Check sheet for the modelled part. Datum: model origin and axes. Units: mm. A direction names the side the tool comes from. Give positions to 0.01 mm unless a question says otherwise; leave off trailing zeros. Order: outer loops, then holes, each group sorted by start corner. A loop starts at its lowest first (then second) coordinate and runs counter-clockwise, first axis right, second up. Notation, with made-up numbers: M 4,33 L 27,33 A16 cw 27,56 Z; hole C -24.75,34.5 d11. An arc over 180 degrees is marked long. Return JSON: item names as keys, results as strings. Group by question number.
Autodesk Inventor part; units mm, degrees
ref_plane "YZ Plane" through (0, 0, 0) normal (1, 0, 0) x (0, 1, 0)
ref_plane "XZ Plane" through (0, 0, 0) normal (0, 1, 0) x (-1, 0, 0)
ref_plane "XY Plane" through (0, 0, 0) normal (0, 0, 1) x (1, 0, 0)
sketch "Sketch51" plane through (0, 0, 0) normal (0, 1, 0) x (-1, 0, 0)
  line L0 (1.3484, 37.0338) -> (-3.7316, 37.0338)
  line L1 (-3.7316, 37.0338) -> (-3.7316, -191.5662)
  line L2 (-3.7316, -191.5662) -> (1.3484, -191.5662)
  line L3 (1.3484, -191.5662) -> (1.3484, 37.0338)
  point P0 (0, 0)
  dimension "d172" = 5.08
  dimension "d173" = 228.6
extrude "Extrusion37" add sketch "Sketch51" along normal blind 71.12
sketch "Sketch52" plane through (-1.3484, 0, 37.0338) normal (0, 0, 1) x (1, 0, 0)
  line L0 (5.08, 0) -> (5.08, 71.12)
  line L1 (5.08, 71.12) -> (-24.13, 71.12)
  line L2 (-24.13, 71.12) -> (-24.13, 66.04)
  line L3 (-24.13, 66.04) -> (5.08, 66.04)
  line L4 (5.08, 66.04) -> (5.08, 71.12)
  point P0 (1.3484, 0)
  dimension "d176" = 5.08
  dimension "d177" = 29.21
extrude "Extrusion38" add sketch "Sketch52" against normal blind 228.6
sketch "Sketch54" plane through (0, 0, 0) normal (0, -1, 0) x (1, 0, 0)
  line L0 (-20.3984, 37.0338) -> (-141.0484, 37.0338)
  line L1 (-141.0484, 37.0338) -> (-141.0484, -191.5662)
  line L2 (-141.0484, -191.5662) -> (-20.3984, -191.5662)
  line L3 (-20.3984, -191.5662) -> (-20.3984, 37.0338)
  line L4 (-25.4784, 37.0338) -> (-1.3484, 37.0338)
  line L5 (-1.3484, -191.5662) -> (-25.4784, -191.5662)
  line L6 (-1.3484, -191.5662) -> (-1.3484, 37.0338)
  point P0 (0, 0)
  dimension "d180" = 0
  dimension "d181" = 0
  dimension "d182" = 19.05
  dimension "d183" = 120.65
extrude "Extrusion39" add sketch "Sketch54" against normal blind 5.08 contours L3 L2 L1 L0
sketch "Sketch55" plane through (-1.3484, 0, 37.0338) normal (0, 0, 1) x (1, 0, 0)
  line L0 (-139.7, 5.08) -> (-19.05, 5.08)
  line L1 (-24.13, 66.04) -> (-24.13, 71.12)
  line L2 (-19.05, 5.08) -> (-24.13, 5.08)
  line L3 (-24.13, 5.08) -> (-24.13, 71.12)
  line L4 (-24.13, 71.12) -> (-19.05, 71.12)
  line L5 (-19.05, 71.12) -> (-19.05, 5.08)
  point P0 (1.3484, 0)
extrude "Extrusion40" add sketch "Sketch55" against normal blind 228.6
sketch "Sketch56" plane through (3.7316, 0, 37.0338) normal (0, 0, 1) x (1, 0, 0)
  line L0 (-29.4089, 71.1531) -> (0, 71.1531)
  line L1 (0, 71.1531) -> (0, 0)
  line L2 (0, 0) -> (-29.4089, 0)
  line L3 (-29.4089, 0) -> (-29.4089, 71.1531)
  point P0 (-3.7316, 0)
extrude "Extrusion41" add sketch "Sketch56" against normal blind 5.08
sketch "Sketch57" plane through (3.7316, 0, -191.5662) normal (0, 0, -1) x (-1, 0, 0)
  line L0 (29.4089, 5.08) -> (29.4089, 71.1531)
  line L1 (29.4089, 71.1531) -> (0, 71.1531)
  line L2 (0, 71.1531) -> (0, 0)
  line L3 (0, 0) -> (29.4089, 0)
  line L4 (29.4089, 0) -> (29.4089, 71.1531)
  point P0 (3.7316, 0)
extrude "Extrusion42" add sketch "Sketch57" against normal blind 5.08
sketch "Sketch58" plane through (0, 71.12, 0) normal (0, 1, 0) x (1, 0, 0)
  line L0 (-25.4784, -31.9538) -> (-25.4784, 186.4862)
  line L1 (-141.0484, 191.5662) -> (-141.0484, -37.0338)
  line L2 (-25.4784, 109.0162) -> (-141.0484, 109.0162)
  line L3 (-141.0484, 109.0162) -> (-141.0484, 147.1162)
  line L4 (-141.0484, 147.1162) -> (-25.4784, 147.1162)
  line L5 (-25.4784, 147.1162) -> (-25.4784, 109.0162)
  line L6 (-25.6773, 191.5662) -> (-141.0484, 191.5662)
  point P0 (0, 0)
  dimension "d192" = 38.1
  dimension "d193" = 44.45
extrude "Extrusion43" add sketch "Sketch58" against normal blind 5.08
sketch "Sketch59" plane through (-141.0484, 71.12, -147.1162) normal (-1, 0, 0) x (0, 0, 1)
  line L0 (0, 0) -> (0, -5.08)
  line L1 (184.15, -71.12) -> (-44.45, -71.12)
  line L2 (0, 0) -> (5.08, 0)
  line L3 (5.08, 0) -> (5.08, -71.12)
  line L4 (5.08, -71.12) -> (0, -71.12)
  line L5 (0, -71.12) -> (0, 0)
  line L6 (38.1, 0) -> (38.1, -5.08)
  line L7 (38.1, 0) -> (33.02, 0)
  line L8 (33.02, 0) -> (33.02, -71.12)
  line L9 (33.02, -71.12) -> (38.1, -71.12)
  line L10 (38.1, -71.12) -> (38.1, 0)
  point P0 (147.1162, -71.12)
  dimension "d196" = 5.08
  dimension "d197" = 5.08
extrude "Extrusion44" add sketch "Sketch59" against normal blind 120.65
sketch "Sketch60" plane through (-141.0484, 0, -191.5662) normal (-1, 0, 0) x (0, 0, 1)
  line L0 (49.53, 5.08) -> (77.47, 5.08)
  line L1 (5.08, 0) -> (223.52, 0)
  line L2 (49.53, 5.08) -> (77.4104, 5.08)
  line L3 (77.4104, 5.08) -> (77.4104, 0)
  line L4 (77.4104, 0) -> (49.53, 0)
  line L5 (49.53, 0) -> (49.53, 5.08)
  point P0 (191.5662, 0)
extrude "Extrusion45" cut sketch "Sketch60" against normal blind 120.65
sketch "Sketch61" plane through (-25.4784, 66.04, -142.0362) normal (-1, 0, 0) x (0, 0, 1)
  line L0 (0, -66.04) -> (0, 0)
  line L1 (27.94, 0) -> (27.94, -60.96)
  line L2 (27.94, 0) -> (0, 0)
  line L3 (-44.45, -66.04) -> (173.99, -66.04)
  line L4 (0, 0) -> (27.6512, 0)
  line L5 (27.6512, 0) -> (27.6512, -66.04)
  line L6 (27.6512, -66.04) -> (0, -66.04)
  line L7 (0, -66.04) -> (0, 0)
  point P0 (142.0362, -66.04)
extrude "Extrusion46" cut sketch "Sketch61" against normal blind 5.08
sketch "Sketch62" plane through (-141.0484, 5.08, -109.0162) normal (-1, 0, 0) x (0, 0, 1)
  line L0 (-33.02, -5.08) -> (-82.55, -5.08)
  line L1 (-38.1, 66.04) -> (-38.1, 0)
  line L2 (0, 66.04) -> (0, 0)
  line L3 (-5.1396, 0) -> (-5.1396, -5.08)
  line L4 (146.05, -5.08) -> (-5.1396, -5.08)
  line L5 (146.05, -5.08) -> (146.05, 0)
  line L6 (0, 0) -> (146.05, 0)
  line L7 (0, 66.04) -> (0, 0)
  line L8 (0, 66.04) -> (-38.1, 66.04)
  line L9 (-38.1, 66.04) -> (-38.1, 0)
  line L10 (-82.55, 0) -> (-38.1, 0)
  line L11 (-82.55, -5.08) -> (-82.55, 0)
  line L12 (-33.02, -5.08) -> (-82.55, -5.08)
  line L13 (-33.02, -5.08) -> (-33.02, 60.96)
  line L14 (-5.08, 60.96) -> (-33.02, 60.96)
  line L15 (-5.08, 60.96) -> (-5.08, 0)
  line L16 (0, 66.04) -> (-34.1859, 66.04)
  line L17 (-34.1859, 66.04) -> (-34.1859, -5.08)
  line L18 (-34.1859, -5.08) -> (0, -5.08)
  line L19 (0, -5.08) -> (0, 66.04)
  line L20 (-5.1396, 0) -> (-5.08, 0)
  point P0 (109.0162, -5.08)
extrude "Extrusion47" add sketch "Sketch62" against normal blind 5.08 contours L0 L17 L8 L2 L19 L4 L3 L20 L15 L14 L13 | L13 L14 L15 L20 L3 L18
sketch "Sketch63" plane through (3.7316, 0, -191.5662) normal (0, 0, -1) x (-1, 0, 0)
  line L0 (0, 0) -> (144.78, 0)
  line L1 (29.4089, 5.08) -> (29.4089, 71.1531)
  point P0 (3.7316, 0)
  point P1 (14.1689, 25.4)
  dimension "d206" = 25.4
  dimension "d207" = 15.24
hole "Hole8" at (-10.4373, 25.4, -191.5662) direction (0, 0, 1) diameter 3.302 end through all
sketch "Sketch64" plane through (-141.0484, 0, -191.5662) normal (-1, 0, 0) x (0, 0, 1)
  line L0 (228.6, 0) -> (0, 0)
  line L1 (44.45, 71.12) -> (44.45, 5.08)
  point P0 (191.5662, 0)
  point P1 (63.5, 25.4)
  dimension "d215" = 25.4
  dimension "d216" = 19.05
hole "Hole9" at (-141.0484, 25.4, -128.0662) direction (1, 0, 0) diameter 3.302 depth 25.4 tip angle 118.188
sketch "Sketch66" plane through (0, 71.12, 0) normal (0, 1, 0) x (1, 0, 0)
  line L0 (-141.0484, 109.0162) -> (-141.0484, 147.1162)
  line L1 (-25.4784, 109.0162) -> (-141.0484, 109.0162)
  line L2 (-141.0484, 147.1162) -> (-25.4784, 147.1162)
  point P0 (0, 0)
  point P1 (-77.5484, 137.5912)
  point P2 (-77.5484, 118.5412)
  dimension "d224" = 0
  dimension "d225" = 63.5
  dimension "d226" = 9.525
  dimension "d227" = 9.525
hole "Hole10" at (-77.5484, 71.12, -137.5912) at (-77.5484, 71.12, -118.5412) direction (0, -1, 0) diameter 3.81 depth 25.4 tip angle 118.188
sketch "Sketch67" plane through (0, 71.12, 0) normal (0, 1, 0) x (1, 0, 0)
  line L0 (-25.4784, -31.9538) -> (-25.4784, 109.0162)
  line L1 (-25.6773, -37.0338) -> (3.7316, -37.0338)
  point P0 (0, 0)
  point P1 (-10.8734, -24.3338)
  point P2 (-10.8734, 51.8662)
  dimension "d235" = 0
  dimension "d236" = 76.2
  dimension "d237" = 14.605
  dimension "d238" = 12.7
hole "Hole11" at (-10.8734, 71.12, 24.3338) at (-10.8734, 71.12, -51.8662) direction (0, -1, 0) diameter 3.81 depth 25.4 tip angle 118.188
sketch "Sketch68" plane through (-141.0484, 71.12, -109.0162) normal (0, 0, 1) x (1, 0, 0)
  line L0 (50.8, -38.1) -> (76.2, -38.1) construction
  line L1 (50.8, -63.5) -> (76.2, -63.5)
  line L2 (76.2, -12.7) -> (50.8, -12.7)
  arc A0 (50.8, -12.7) -> (50.8, -63.5) centre (50.8, -38.1) ccw
  arc A1 (76.2, -63.5) -> (76.2, -12.7) centre (76.2, -38.1) ccw
  line L3 (115.57, 0) -> (0, 0)
  line L4 (0, 0) -> (0, -66.04)
  point P0 (141.0484, -71.12)
  point P1 (63.5, -38.1)
  dimension "d246" = 38.1
  dimension "d247" = 25.4
  dimension "d248" = 50.8
  dimension "d249" = 25.4
extrude "Extrusion48" cut sketch "Sketch68" against normal blind 77.7875
equation "\"d172\" = WallWidth"
equation "\"d173\" = PartLength"
equation "\"d174\" = CPDeckHeight"
equation "\"d176\" = WallWidth"
equation "\"d177\" = 2 * WallWidth + ControlPlateShelfLength"
equation "\"d178\" = PartLength"
equation "\"d182\" = ControlPlateShelfLength"
equation "\"d183\" = CPDWidthHole"
equation "\"d184\" = WallWidth"
equation "\"d186\" = PartLength"
equation "\"d188\" = WallWidth"
equation "\"d190\" = WallWidth"
equation "\"d194\" = WallWidth"
equation "\"d196\" = WallWidth"
equation "\"d197\" = WallWidth"
equation "\"d202\" = WallWidth"
equation "\"d204\" = WallWidth"
equation "\"DSLength\" = 1371.6"
equation "\"DSWidth\" = 304.8"
equation "\"DCDeckHeight\" = 76.2"
equation "\"WallWidth\" = 5.08"
equation "\"EdgeAngle\" = 10deg"
equation "\"LengthCuts\" = 152.4"
equation "\"WidthCuts\" = 50.8"
equation "\"PartLength\" = 228.6"
equation "\"PartWidth\" = 152.4"
equation "\"BoltHoldDiam\" = 6.35"
equation "\"ControlPlateLength\" = 228.6"
equation "\"ControlPlateWidth\" = 228.6"
equation "\"ControlPlateShelfLength\" = 19.05"
equation "\"ControlHoleLength\" = 190.5"
equation "\"ControlHoleWidth\" = 190.5"
equation "\"ControlHoleFromSide\" = 63.5"
equation "\"ControlHoleBoltHoleMid\" = 9.525"
equation "\"CPDeckHeight\" = 71.12"
equation "\"CPFromSide\" = 63.5"
equation "\"CPFromBack\" = 63.5"
equation "\"DU1CHWidth\" = 69.85"
equation "\"DU1CHLength\" = 146.05"
equation "\"ControlPlateScrewLength\" = 76.2"
equation "\"DSBackHeight\" = 127"
equation "\"BackShelf\" = 25.4"
equation "\"MainAngle\" = 168.22deg"
equation "\"CPDWidthHole\" = 120.65"
equation "\"CPDLengthHole\" = 146.05"
equation "\"DownBackHeight\" = 130.7084"
properties part number "CPLRightTwo"
1) Sectioned sample at A-A on x = -87. Record the boundary of the cut face in (y, z).
2) Tool access check on faces 1 (the face through (-78, 7.62, -145)), 2 (the face through (-11, 33, -186.486)), 3 (the face through (-25.478, 38, -167)), 4 (the face through (-84, 0, -76)). Record the directions out of +Z, -Z, +X, -X, +Y, -Y that give a thin tool (end or side, any length) a straight path to the whole face; none if there is none.
3) Material ranges on line 1 along Z through (x, y) = (-9.5, 42); line 2 along X through (y, z) = (4, -74); line 3 along Z through (x, y) = (-38, 64), recorded low to high.
4) Sectioned sample at D-D on z = -176. Record the boundary of the cut face in (x, y), then the cut area to 3 significant figures.
5) Sectioned sample at B-B on y = 62. Record the boundary of the cut face in (x, z) (3 decimals), then the cut area to 3 significant figures.
6) Depth check by flat-ended pin: P1, Ø8, axis at x = -71.5, y = 51, coming from the +Z side; P2, Ø5, axis at x = -35.5, y = 51, coming from the +Z side; P3, Ø5, axis at y = 62.5, z = -24.5, coming from the -X side. Enter the tip coordinate at first touch or a pass-through.
7) Release check for a two-part mould opening along X. For faces 5 (the face through (-11, 71.153, 35)), 6 (the face through (-25.677, 38, -189)), 7 (the face through (-77, 58.42, -145)), 8 (the face through (-39.455, 32.461, -111.521)) record: released by +X, released by -X, zero draft, split by the parting line, or undercut.
Reply:
{
 "1": {"outline": "M 0,-191.57 L 5.08,-191.57 L 5.08,-147.12 L 7.62,-147.12 L 7.62,-142.04 L 0,-142.04 Z; M 0,-114.16 L 5.08,-114.16 L 5.08,-114.1 L 7.62,-114.1 L 7.62,-109.02 L 5.08,-109.02 L 5.08,37.03 L 0,37.03 Z; M 58.42,-147.12 L 71.12,-147.12 L 71.12,-109.02 L 58.42,-109.02 L 58.42,-114.1 L 66.04,-114.1 L 66.04,-142.04 L 58.42,-142.04 Z"},
 "2": {"face 1": "+Z, -Z", "face 2": "-Y", "face 3": "-X, +Y", "face 4": "+Z, -Z, +X, -X, -Y"},
 "3": {"line 1": "-191.57 to -186.49, 31.95 to 37.03", "line 2": "-141.05 to -20.4, -1.35 to 3.73", "line 3": "-147.12 to -142.04, -114.1 to -109.02"},
 "4": {"outline": "M -141.05,0 L -20.4,0 L -20.4,66.04 L -1.35,66.04 L -1.35,0 L 3.73,0 L 3.73,71.12 L -25.48,71.12 L -25.48,5.08 L -141.05,5.08 Z", "area": "1,410 mm^2"},
 "5": {"outline": "M -141.048,-147.116 L -25.478,-147.116 L -25.478,-186.486 L -25.677,-186.486 L -25.677,-191.566 L 3.732,-191.566 L 3.732,37.034 L -25.677,37.034 L -25.677,31.954 L -25.478,31.954 L -25.478,-109.016 L -141.048,-109.016 Z; hole M -135.968,-142.036 L -20.398,-142.036 L -20.398,-186.486 L -1.348,-186.486 L -1.348,31.954 L -20.398,31.954 L -20.398,-114.385 L -25.478,-114.385 L -25.478,-114.096 L -135.968,-114.096 Z", "area": "3,690 mm^2"},
 "6": {"P1": "through", "P2": "z = -109.02", "P3": "x = -25.48"},
 "7": {"face 5": "zero draft", "face 6": "released by -X", "face 7": "undercut", "face 8": "undercut"}
}
